For this review, take the finished solid that the model builds, in its own axes (mm). Face numbers are marked on the shaded views. Give positions to 0.01 mm unless a question says otherwise; leave off trailing zeros. Write each loop counter-clockwise with the first axis right and the second up, starting at its lowest first coordinate (ties: lowest second). Pieces come first, ordered by that corner, then holes.
1) We need section A-A on y = 0. Give the boundary of the cut face in (x, z), and give its area (3 significant figures).
2) We need section B-B on x = -34.5. Give the boundary of the cut face in (y, z).
3) Draft analysis for pull direction Y (two halves, no side actions). For the marked faces 1, 2 and 3, state which applies: pulls with the +Y half, pulls with the -Y half, needs draft (parallel to the pull), parting line crosses it, or undercut.
4) For P1, Ø3, axis at y = -22.62, z = 15.88, coming from the +X side; P2, Ø10, axis at y = -18.5, z = 18, coming from the +X side; P3, Ø10, axis at y = 22.5, z = 12.5, coming from the -X side; P4, Ø1.1, axis at y = 0, z = 22, coming from the +X side, all flat-tipped, find the tip position at first contact; note any pin that passes through.
5) Wall thickness on line 1 along Y through (x, z) = (-51.5, 10); line 2 along Y through (x, z) = (-50.5, 10.5); line 3 along X through (y, z) = (29, 16): over which ranges is each line inside the solid? List them lowest first.
6) We need section D-D on y = 33. Give the boundary of the cut face in (x, z), and give its area (3 significant figures).
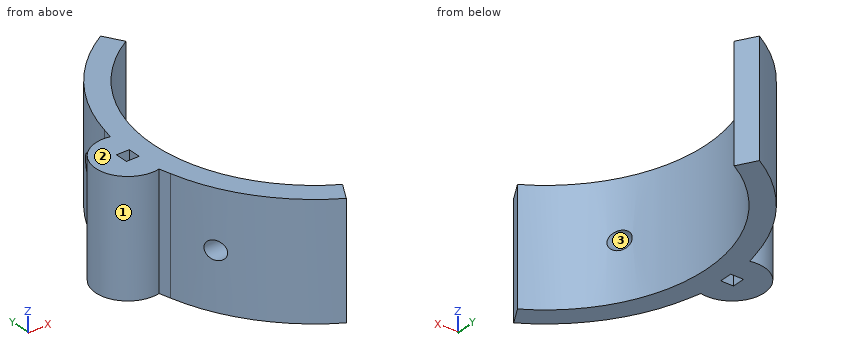
from build123d import *

# Parameters (mm, degrees)
F0_R     = 1.27
F1_DEPTH = 31.75
F2_W     = 3.556
F2_H     = 3.556
F2_R     = 1.27
F3_DEPTH = 31.75
F5_D     = 5.1054


with BuildPart() as f1:
    # F0 (on Top) → F1 (new body)
    with BuildSketch(Plane.XY):
        with BuildLine():
            ThreePointArc((-22.225, -38.494829), (-44.45, 0), (-22.225, 38.494829))
            Line((-22.225, 38.494829), (-25.2095, 43.664135))
            ThreePointArc((-25.2095, 43.664135), (-40.403306, 30.160378), (-49.029733, 11.754185))
            Line((-49.029733, 11.754185), (-49.807311, 8.688576))
            ThreePointArc((-49.807311, 8.688576), (-60.579, 0), (-49.807311, -8.688576))
            Line((-49.807311, -8.688576), (-49.029733, -11.754185))
            ThreePointArc((-49.029733, -11.754185), (-40.403306, -30.160378), (-25.2095, -43.664135))
            Line((-25.2095, -43.664135), (-22.225, -38.494829))
        make_face()
        with Locations((-51.689, 0)):
            Circle(F0_R, mode=Mode.SUBTRACT)
    extrude(amount=F1_DEPTH)

    # F2 (on face) → F3 (cut, through all)
    with BuildSketch(Plane.XY.offset(31.75)):
        with Locations((-51.689, 0)):
            Rectangle(F2_W, F2_H)
        with Locations((-51.689, 0)):
            Circle(F2_R, mode=Mode.SUBTRACT)
    extrude(amount=-F3_DEPTH, mode=Mode.SUBTRACT)

    # F5 (through all)
    with Locations(Plane.YZ):
        with Locations((-22.624822, 15.875), (23.095178, 15.875)):
            Hole(F5_D / 2)


solid = f1.part
Results list:
1. outline: (-60.58, 0) - (-53.47, 0) - (-53.47, 31.75) - (-60.58, 31.75) - close; (-49.91, 0) - (-44.45, 0) - (-44.45, 31.75) - (-49.91, 31.75) - close
1. area: 399 mm2
2. outline: (-36.77, 0) - (-28.03, 0) - (-28.03, 31.75) - (-36.77, 31.75) - close; (28.03, 0) - (36.77, 0) - (36.77, 31.75) - (28.03, 31.75) - close
3. face 1: parting line crosses it
3. face 2: needs draft
3. face 3: undercut
4. P1: passes through
4. P2: stops at x = -37.73
4. P3: stops at x = -47.28
4. P4: stops at x = -44.45
5. line 1: y = -8.89 to -1.78, 1.78 to 8.89
5. line 2: y = -8.81 to -1.78, 1.78 to 8.81
5. line 3: x = -41.24 to -33.69
6. outline: (-38.12, 0) - (-29.78, 0) - (-29.78, 31.75) - (-38.12, 31.75) - close
6. area: 265 mm2
